Can you work these out from the model? Positions are in its coordinate system, mm. Face numbers are marked on the shaded views. A direction names the side the tool comes from. Round coordinates to 2 decimals unless told otherwise and drop trailing zeros. Write each loop counter-clockwise with the first axis right and the second up, starting at its lowest first coordinate (ties: lowest second). Pieces come first, ordered by that corner, then holes. Notation, with made-up numbers: (14.25, 7.5) - (67.25, 7.5) arc R10 ccw to (67.25, 12.5) - close; hole circle Ø3 at (62.5, -13). An arc over 180 degrees is marked (long way). One line per item, written item: value. Start each with the question number.
(1) I'm going to push flat-ended pins straight in: pin 1 Ø1.5 at (y, z) = (110.5, 183.5) entering from -X; pin 2 Ø3 at (y, z) = (122.5, 198) entering from -X; pin 3 Ø10 at (y, z) = (109, 182.5) entering from +X; pin 4 Ø6 at (x, z) = (-3.5, 195) entering from +Y. Where does each tip first touch, or does it pass through?
(2) I want a section at D-D on z = 182.5. List the corners of the cut face in (x, y) for me, plus the area to 3 significant figures.
(3) If I drill on L1, parallel to X at y = 118.5, z = 175; L2, parallel to X at y = 105.3, z = 199; L3, parallel to X at y = 130.3, z = 199.5, over which ranges is the centre line in solid material (lowest first)? Write a range as from..to.
(4) I want a section at B-B on x = -22.5. List the corners of the cut face in (y, z) for me.
(5) I want a section at C-C on y = 105. List the corners of the cut face in (x, z) for me, plus the area to 3 significant figures.
(6) On a 3-axis mill with a long thin cutter (end or side, diameter ignored), from which of +Z, -Z, +X, -X, +Y, -Y can I reach the whole of each face in a straight line? I mean the marked faces 1, 2, 3 and 4. Say none if no direction works.
(7) I want a section at A-A on y = 127.5. Give the number of separate pieces and of enclosed holes in the cut face, plus the area to 3 significant figures.
(8) Thinking about a two-plate mould opening in Z: for the marked faces 5, 6 and 7, which applies, +Z half, -Z half, draft (parallel to the pull), parting line (faces both ways), or undercut?
from build123d import *

# Parameters (mm, degrees)
SKETCH088_W     = 38
SKETCH088_H     = 31
PAD029_DEPTH    = 30
POCKET029_DEPTH = 31.001
SKETCH100_R     = 14
POCKET030_DEPTH = 30.001
SKETCH101_W     = 25
SKETCH101_H     = 10
POCKET031_DEPTH = 3
SKETCH102_R     = 2.3
POCKET032_DEPTH = 5.5
SKETCH103_W     = 6
SKETCH103_H     = 31
PAD035_DEPTH    = 6
POCKET033_DEPTH = 30.001
PAD037_DEPTH    = 6
SKETCH107_R     = 1.7
HOLE020_DEPTH   = 25


with BuildPart() as part:
    # Sketch088 → Pad029 (new body)
    with BuildSketch(Plane.XZ.offset(3)):
        with Locations((0, 187.5)):
            Rectangle(SKETCH088_W, SKETCH088_H)
    extrude(amount=-PAD029_DEPTH)

    # Sketch099 (on Face4 of Pad029) → Pocket029 (cut, through all)
    with BuildSketch(Plane(origin=(0, 0, 203), x_dir=(-1, 0, 0), z_dir=(0, 0, 1))):
        with BuildLine():
            Line((-12.5, -14), (-12.5, -24))
            Line((-12.5, -24), (12.5, -24))
            Line((12.5, -14), (12.5, -24))
            ThreePointArc((12.5, -14), (0, -1.5), (-12.5, -14))
        make_face()
    extrude(amount=-POCKET029_DEPTH, mode=Mode.SUBTRACT)

    # Sketch100 (on Face4 of Pocket029) → Pocket030 (cut, through all)
    with BuildSketch(Plane.XZ.offset(3)):
        with Locations((0, 187)):
            Circle(SKETCH100_R)
    extrude(amount=-POCKET030_DEPTH, mode=Mode.SUBTRACT)

    # Sketch101 (on Face5 of Pocket030) → Pocket031 (cut)
    with BuildSketch(Plane(origin=(0, 27, 0), x_dir=(1, 0, 0), z_dir=(0, 1, 0))):
        with Locations((0, -177)):
            Rectangle(SKETCH101_W, SKETCH101_H)
    extrude(amount=-POCKET031_DEPTH, mode=Mode.SUBTRACT)

    # Sketch102 (on Face4 of Pocket031) → Pocket032 (cut)
    with BuildSketch(Plane.XZ.offset(3)):
        with Locations((-12, 199)):
            Circle(SKETCH102_R)
        with Locations((-12, 175)):
            Circle(SKETCH102_R)
        with Locations((12, 175)):
            Circle(SKETCH102_R)
        with Locations((12, 199)):
            Circle(SKETCH102_R)
    extrude(amount=-POCKET032_DEPTH, mode=Mode.SUBTRACT)

    # Sketch103 → Pad035 (join)
    with BuildSketch(Plane.XZ.offset(-27)):
        with Locations((-23, 187.5)):
            Rectangle(SKETCH103_W, SKETCH103_H)
        with Locations((23, 187.5)):
            Rectangle(SKETCH103_W, SKETCH103_H)
    extrude(amount=PAD035_DEPTH)

    # Sketch104 → Pocket033 (cut, through all)
    with BuildSketch(Plane.XZ.offset(-27)):
        Polygon((-26, 197.999996), (-15, 187), (-15, 172), (-26, 172), align=None)
        Polygon((26, 197.999996), (15, 187), (15, 172), (26, 172), align=None)
    extrude(amount=POCKET033_DEPTH, mode=Mode.SUBTRACT)

    # Sketch106 → Pad037 (join)
    with BuildSketch(Plane.XZ.offset(-27)):
        Polygon((-19, 203), (-26, 203), (-26, 198), (-19, 191), align=None)
        Polygon((19, 203), (26, 203), (26, 198), (19, 191), align=None)
    extrude(amount=PAD037_DEPTH)

    # Sketch107 (on Face4 of Pad037) → Hole020 (cut)
    with BuildSketch(Plane.XZ.offset(-21)):
        with Locations((-22.5, 199.5)):
            Circle(SKETCH107_R)
        with Locations((22.5, 199.5)):
            Circle(SKETCH107_R)
    extrude(amount=-HOLE020_DEPTH, mode=Mode.SUBTRACT)


with BuildPart() as part_1:
    # Body012 placement: moved
    add(part.part.moved(Location((0, 105, 0))))


solid = part_1.part
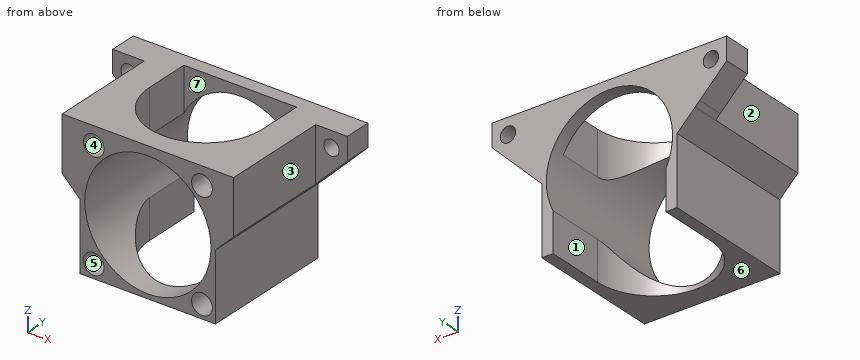
Established:
1. pin 1: x = -15
1. pin 2: x = -19
1. pin 3: x = 15.5
1. pin 4: through
2. outline: (-15, 102) - (-13.26, 102) - (-13.26, 132) - (-15, 132) - close; (13.26, 102) - (15, 102) - (15, 132) - (13.26, 132) - close
2. area: 105 mm2
3. L1: -15..-12.49, 12.49..15
3. L2: -19..-14.3, -9.7..-7.21, 7.21..9.7, 14.3..19
3. L3: -26..-24.2, -20.8..-6.3, 6.3..20.8, 24.2..26
4. outline: (126, 194.5) - (132, 194.5) - (132, 197.8) - (126, 197.8) - close; (126, 201.2) - (132, 201.2) - (132, 203) - (126, 203) - close
5. outline: (-19, 191) - (-15, 187) - (-15, 172) - (15, 172) - (15, 187) - (19, 191) - (19, 203) - (-19, 203) - close; hole circle Ø4.6 at (-12, 175); hole circle Ø4.6 at (-12, 199); hole circle Ø28 at (0, 187); hole circle Ø4.6 at (12, 175); hole circle Ø4.6 at (12, 199)
5. area: 360 mm2
6. face 1: -Z, +Y
6. face 2: +Z, -Z, -X, -Y
6. face 3: +Z, -Z, +X, -Y
6. face 4: -Y
7. separate pieces: 2
7. enclosed holes: 2
7. area: 342 mm2
8. face 5: undercut
8. face 6: -Z half
8. face 7: draft
